Autodesk Fusion 360 part; units mm, degrees
sketch "Sketch1" plane through (0, 0, 0) normal (0, 1, 0) x (1, 0, 0)
  line L0 (0, -25.4) -> (0, 0)
  line L1 (0, 0) -> (25.4, 0)
  line L2 (12.7, -12.7) -> (11.05, -11.05) construction
  line L3 (3.175, -25.4) -> (3.175, -3.175)
  line L4 (3.175, -3.175) -> (25.4, -3.175)
  line L5 (25.4, -3.175) -> (25.4, 0)
  line L6 (0, -25.4) -> (3.175, -25.4)
  dimension "d1" = 25.4
  dimension "d2" = 25.4
  dimension "d13" = 3.175
extrude "Extrude1" add sketch "Sketch1" along normal blind 250
sketch "Sketch2" plane through (3.175, 0, 0) normal (1, 0, 0) x (0, 0, -1)
  line L0 (-25.4, 0) -> (-3.175, 0)
  line L1 (-3.175, 0) -> (-3.175, 250)
  line L2 (-3.175, 250) -> (-25.4, 250)
  line L3 (-25.4, 250) -> (-25.4, 0)
  circle A0 centre (-14.2875, 235.712) radius 2.76
  circle A1 centre (-14.2875, 11.1125) radius 2.5546
  line L4 (-14.2875, 250) -> (-14.2875, 0) construction
  dimension "d14" = 14.288
  dimension "d15" = 11.1125
hole "Hole1" at (3.175, 11.1125, 14.2875) at (3.175, 235.712, 14.2875) direction (-1, 0, 0) diameter 6.5 end through all
hole "Hole2" at (14.287, 210.312, 3.175) direction (0, 0, -1) diameter 6.5 end through all
equation "d15 = ( 22.225 / 2 ) * 1 mm"
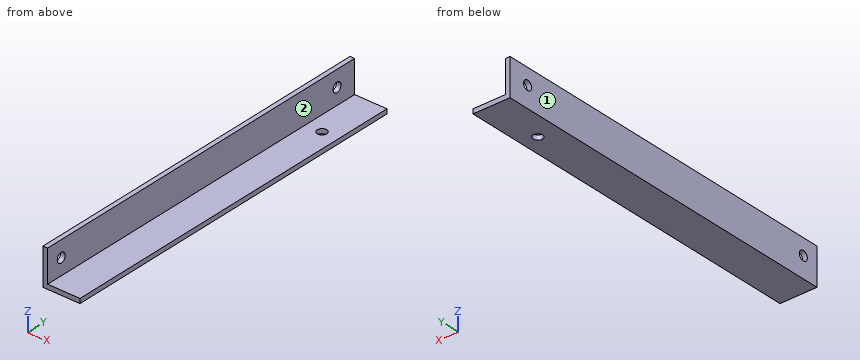
Model file for the job. Use its own axes, mm. Face numbers are marked on the shaded views. A direction names the side the tool comes from. Give positions to 0.01 mm unless a question says otherwise; leave off trailing zeros. Write each loop counter-clockwise with the first axis right and the second up, starting at its lowest first coordinate (ties: lowest second). Pieces come first, ordered by that corner, then holes. Notation, with made-up numbers: (10, -16.5) -> (46, -16.5) arc R19 ccw to (46, 3.5) -> close; hole circle Ø7 at (5.5, 67). An arc over 180 degrees is marked (long way). Write item = value, one per line.
(1) Tool access for the marked faces 1 and 2: list every direction of +Z, -Z, +X, -X, +Y, -Y with a clear straight run to the whole face (end or side of a thin tool).
Determined:
face_1 = +Z, -Z, -X, +Y, -Y
face_2 = +Z, +X, +Y, -Y
(2) Slice it at A-A, the plane z = 15.25. Give the cut face in (x, y) (3 decimals), then the cut area to 3 significant figures.
Determined:
outline = (0, 0) -> (3.175, 0) -> (3.175, 8.008) -> (0, 8.008) -> close; (0, 14.217) -> (3.175, 14.217) -> (3.175, 232.608) -> (0, 232.608) -> close; (0, 238.816) -> (3.175, 238.816) -> (3.175, 250) -> (0, 250) -> close
area = 754 mm2
(3) Slice it at C-C, the plane x = 5.5. Give the cut face in (y, z) (3 decimals).
Determined:
outline = (0, 0) -> (250, 0) -> (250, 3.175) -> (0, 3.175) -> close
(4) Flat gauge pins, fed straight in: P1, Ø11, axis at y = 67, z = 10.5, coming from the +X side (3 decimals); P2, Ø7.5, axis at x = 14.287, y = 210.312, coming from the -Z side; P3, Ø1.5, axis at x = 7, y = 143, coming from the +Z side (3 decimals); P4, Ø5, axis at y = 235.71, z = 14.29, coming from the -X side. Where does each tip first touch, or does it go through?
Determined:
P1 = 3.175
P2 = 0
P3 = 3.175
P4 = through
(5) Probe line 1 along Z through (x, y) = (8.75, 83) (3 decimals); line 2 along Y through (x, z) = (3, 12). List the from-to ranges inside material, lowest first.
Determined:
line_1 = 0 to 3.175
line_2 = 0 to 8.8, 13.42 to 233.4, 238.02 to 250
(6) Slice it at B-B, the plane y = 81. Give the cut face in (x, z) (3 decimals), then the cut area to 3 significant figures.
Determined:
outline = (0, 0) -> (25.4, 0) -> (25.4, 3.175) -> (3.175, 3.175) -> (3.175, 25.4) -> (0, 25.4) -> close
area = 151 mm2
